Design review of the part built by this model. Coordinates are the model's own, in mm. Face numbers are marked on the shaded views. A direction names the side the tool comes from. Give positions to 0.01 mm unless a question says otherwise; leave off trailing zeros. Loops run counter-clockwise (first coordinate to the right, second up) from the corner with the lowest first, then second, coordinate; pieces in that order, holes last. Notation, with made-up numbers: M 5,69 L 50,69 A19 cw 50,100 Z; hole C 33,85 d10. An arc over 180 degrees is marked long. Use CSV: the item, a comma, the result in double quotes.
from build123d import *

# Parameters (mm, degrees)
SKETCH1_W               = 180
SKETCH1_H               = 130
BOSS_EXTRUDE1_DEPTH     = 5
SKETCH2_W               = 70
SKETCH2_H               = 20
CUT_EXTRUDE1_DEPTH      = 2.5
SKETCH3_W               = 65
SKETCH3_H               = 60
SKETCH3_W_2             = 35
SKETCH3_H_2             = 50
CUT_EXTRUDE2_DEPTH      = 2.5
SKETCH4_W               = 30
SKETCH4_H               = 35
SKETCH4_W_2             = 45
SKETCH4_H_2             = 40
SKETCH4_W_3             = 25
CUT_EXTRUDE3_DEPTH      = 2.5
CUT_EXTRUDE3_DEPTH_BACK = 3.5
SKETCH5_W               = 15
SKETCH5_H               = 90
CUT_EXTRUDE4_DEPTH      = 2.5


with BuildPart() as part:
    # Sketch1 → Boss-Extrude1 (new body)
    with BuildSketch(Plane.XY):
        Rectangle(SKETCH1_W, SKETCH1_H)
    extrude(amount=BOSS_EXTRUDE1_DEPTH)

    # Sketch2 → Cut-Extrude1 (cut)
    with BuildSketch(Plane.XY.offset(5)):
        with Locations((-55, 55)):
            Rectangle(SKETCH2_W, SKETCH2_H)
        with Locations((55, 55)):
            Rectangle(SKETCH2_W, SKETCH2_H)
        with Locations((55, -55)):
            Rectangle(SKETCH2_W, SKETCH2_H)
        with Locations((-55, -55)):
            Rectangle(SKETCH2_W, SKETCH2_H)
    extrude(amount=-CUT_EXTRUDE1_DEPTH, mode=Mode.SUBTRACT)

    # Sketch3 → Cut-Extrude2 (cut)
    with BuildSketch(Plane.XY.offset(5)):
        with Locations((-57.5, 0)):
            Rectangle(SKETCH3_W, SKETCH3_H)
        with Locations((2.5, 0)):
            Rectangle(SKETCH3_W_2, SKETCH3_H_2)
        with Locations((47.5, 0)):
            Rectangle(SKETCH3_W_2, SKETCH3_H_2)
    extrude(amount=-CUT_EXTRUDE2_DEPTH, mode=Mode.SUBTRACT)

    # Sketch4 → Cut-Extrude3 (cut, two sides)
    with BuildSketch(Plane.XY.offset(2.5)) as cut_extrude3_sk:
        with Locations((0, 47.5)):
            Rectangle(SKETCH4_W, SKETCH4_H)
        with Locations((0, -47.5)):
            Rectangle(SKETCH4_W, SKETCH4_H)
        with Locations((-57.5, 0)):
            Rectangle(SKETCH4_W_2, SKETCH4_H_2)
        with Locations((47.5, 0)):
            Rectangle(SKETCH4_W_3, SKETCH4_H_2)
        with Locations((2.5, 0)):
            Rectangle(SKETCH4_W_3, SKETCH4_H_2)
    extrude(amount=CUT_EXTRUDE3_DEPTH, mode=Mode.SUBTRACT)
    extrude(cut_extrude3_sk.sketch, amount=-CUT_EXTRUDE3_DEPTH_BACK, mode=Mode.SUBTRACT)

    # Sketch5 → Cut-Extrude4 (cut)
    with BuildSketch(Plane.XY.offset(5)):
        with Locations((82.5, 0)):
            Rectangle(SKETCH5_W, SKETCH5_H)
    extrude(amount=-CUT_EXTRUDE4_DEPTH, mode=Mode.SUBTRACT)


solid = part.part
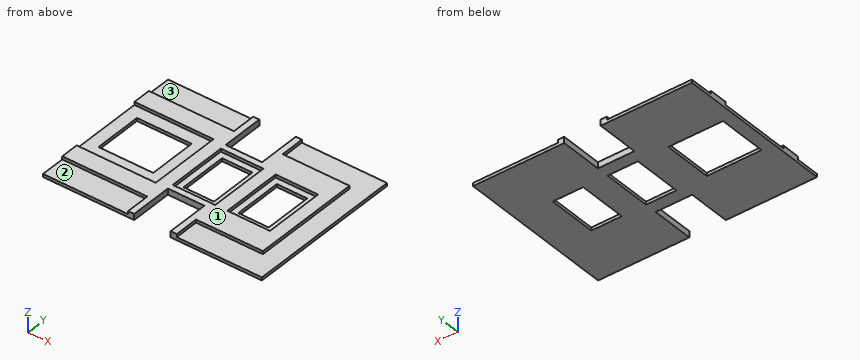
(1) Machinability: for the marked faces 1, 2 and 3, which of the approach directions +Z, -Z, +X, -X, +Y, -Y give a long, thin tool a straight path to every point of the face, cutting with its end or side? Answer none if there is none.
A:
face 1,"+Z, +X, -X, +Y, -Y"
face 2,"+Z, -X, -Y"
face 3,"+Z, -X, +Y"
(2) We need section B-B on y = 54.5. State the section outline as (x, z) points.
A:
outline,"M -90,0 L -15,0 L -15,5 L -20,5 L -20,2.5 L -90,2.5 Z; M 15,0 L 90,0 L 90,2.5 L 20,2.5 L 20,5 L 15,5 Z"
(3) We need section C-C on x = 40.5. State the section outline as (y, z) points, then the cut area to 3 significant figures.
A:
outline,"M -65,0 L -20,0 L -20,2.5 L -25,2.5 L -25,5 L -45,5 L -45,2.5 L -65,2.5 Z; M 20,0 L 65,0 L 65,2.5 L 45,2.5 L 45,5 L 25,5 L 25,2.5 L 20,2.5 Z"
area,"325 mm²"
(4) We need section D-D on x = 17. State the section outline as (y, z) points.
A:
outline,"M -65,0 L 65,0 L 65,5 L 25,5 L 25,2.5 L -25,2.5 L -25,5 L -65,5 Z"
(5) We need section A-A on z = 1.65. State the section outline as (x, y) points, then the cut area to 3 significant figures.
A:
outline,"M -90,-65 L -15,-65 L -15,-30 L 15,-30 L 15,-65 L 90,-65 L 90,65 L 15,65 L 15,30 L -15,30 L -15,65 L -90,65 Z; hole M -80,-20 L -35,-20 L -35,20 L -80,20 Z; hole M -10,-20 L 15,-20 L 15,20 L -10,20 Z; hole M 35,-20 L 60,-20 L 60,20 L 35,20 Z"
area,"17,500 mm²"
(6) Clearance check with flat-ended pins moving along their axes: P1, Ø4, axis at x = 20, y = -4, coming from the -Z side; P2, Ø1.2, axis at y = 8, z = 4, coming from the +X side; P3, Ø8, axis at x = 55.5, y = 3.5, coming from the +Z side; P4, Ø1.2, axis at x = -43, z = 3.5, coming from the +Y side. State where each tip first meets the part, or that it passes through.
A:
P1,"z = 0"
P2,"x = 75"
P3,"through"
P4,"y = 45"
(7) Wall thickness on line 1 along X through (y, z) = (-1.5, 0.9); line 2 along X through (y, z) = (3, 2.7); line 3 along Y through (x, z) = (-12.5, 3): over which ranges is each line inside the solid? List them lowest first. Write a range as [from, to].
A:
line 1,"[-90, -80], [-35, -10], [15, 35], [60, 90]"
line 2,"[-25, -15], [20, 30], [65, 75]"
line 3,"[-30, -25], [25, 30]"
